from build123d import *

# Parameters (mm, degrees)
F0_R     = 1.5
F1_DEPTH = 1
F4_DEPTH = 66.75
F5_DEPTH = 1


with BuildPart() as f1:
    # F0 (on Top) → F1 (new body)
    with BuildSketch(Plane.XY):
        with BuildLine():
            ThreePointArc((-29, 10.75), (-30.767766953, 10.017766953), (-31.5, 8.25))
            Line((-31.5, 8.25), (-31.5, -8.25))
            ThreePointArc((-31.5, -8.25), (-30.767766953, -10.017766953), (-29, -10.75))
            Line((-29, -10.75), (-22.5, -10.75))
            Line((-22.5, -10.75), (-22.5, 10.75))
            Line((-22.5, 10.75), (-29, 10.75))
        make_face()
        with Locations((-27, -7.625)):
            Circle(F0_R, mode=Mode.SUBTRACT)
        with Locations((-27, 7.625)):
            Circle(F0_R, mode=Mode.SUBTRACT)
    extrude(amount=F1_DEPTH)



with BuildPart() as f1b:
    # F0 (on Top) → F1, piece 2 (new body)
    with BuildSketch(Plane.XY):
        with BuildLine():
            Line((29, 10.75), (22.5, 10.75))
            Line((22.5, 10.75), (22.5, -10.75))
            Line((22.5, -10.75), (29, -10.75))
            ThreePointArc((29, -10.75), (30.767766953, -10.017766953), (31.5, -8.25))
            Line((31.5, -8.25), (31.5, 8.25))
            ThreePointArc((31.5, 8.25), (30.767766953, 10.017766953), (29, 10.75))
        make_face()
        with Locations((27, -7.625)):
            Circle(F0_R, mode=Mode.SUBTRACT)
        with Locations((27, 7.625)):
            Circle(F0_R, mode=Mode.SUBTRACT)
    extrude(amount=F1_DEPTH)


with BuildPart() as f1_1:
    add(f1.part)

    add(f1b.part)  # F4 merges F1b
    # F3 (on offset) → F4 (join)
    with BuildSketch(Plane(origin=(0, 0, -11.5), x_dir=(1, 0, 0), z_dir=(0, 0, -1))):
        Polygon((-22.5, 10.75), (-22.5, -10.75), (-22.5, -15.75), (22.5, -15.75), (22.5, -10.75), (22.5, 10.75), (22.5, 15.75), (-22.5, 15.75), align=None)
        Polygon((-21.5, -14.75), (-21.5, -10.75), (-21.5, 10.75), (-21.5, 14.75), (21.5, 14.75), (21.5, 10.75), (21.5, -10.75), (21.5, -14.75), (8, -14.75), (-8, -14.75), align=None, mode=Mode.SUBTRACT)
    extrude(amount=-F4_DEPTH)

    # F3 (on offset) → F5 (join)
    with BuildSketch(Plane(origin=(0, 0, -11.5), x_dir=(1, 0, 0), z_dir=(0, 0, -1))):
        with BuildLine():
            Line((-21.5, 10.75), (-21.5, -10.75))
            Line((-21.5, -10.75), (-21.5, -14.75))
            Line((-21.5, -14.75), (-8, -14.75))
            Line((-8, -14.75), (-8, 0))
            ThreePointArc((-8, 0), (0, 8), (8, 0))
            Line((8, 0), (8, -14.75))
            Line((8, -14.75), (21.5, -14.75))
            Line((21.5, -14.75), (21.5, -10.75))
            Line((21.5, -10.75), (21.5, 10.75))
            Line((21.5, 10.75), (21.5, 14.75))
            Line((21.5, 14.75), (-21.5, 14.75))
            Line((-21.5, 14.75), (-21.5, 10.75))
        make_face()
    extrude(amount=-F5_DEPTH)


solid = f1_1.part
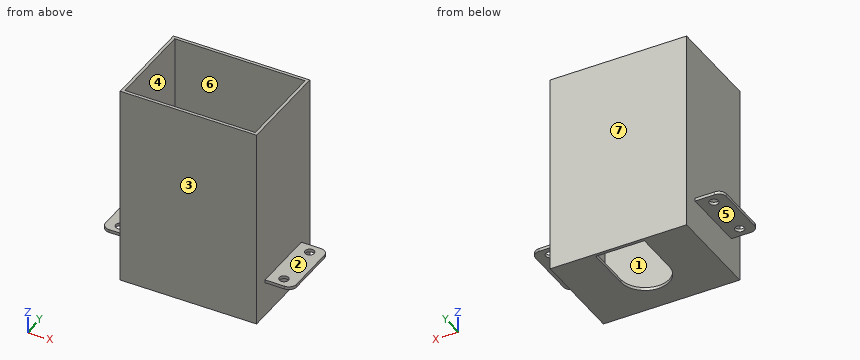
Source: CAD feature listing. Evaluate the final solid. Frame: model axes, mm. Face numbers are marked on the shaded views. A direction names the side the tool comes from. Coordinates: 2 decimals unless noted, no trailing zeros. Loops run counter-clockwise (first coordinate to the right, second up) from the corner with the lowest first, then second, coordinate; pieces in that order, holes last. Notation, with made-up numbers: (68.25, -18.5) - (111.25, -18.5) arc R22 cw to (111.25, 8.5) - close; hole circle Ø3 at (41, 9). An arc over 180 degrees is marked (long way). Return JSON: item names as keys, results as strings.
Q1. Material intervals for line 1 along Y through (x, z) = (27, 0.3) (3 decimals); line 2 along Y through (x, z) = (18.5, 26.5); line 3 along X through (y, z) = (-11.5, 35.5), sorted ascending.
Results:
{"line 1": "-10.75 to -9.125, -6.125 to 6.125, 9.125 to 10.75", "line 2": "-15.75 to -14.75, 14.75 to 15.75", "line 3": "-22.5 to -21.5, 21.5 to 22.5"}
Q2. Contact query for flat-ended pins moving along their axis: P1, Ø7, axis at x = 28.5, y = 3.5, coming from the -Z side; P2, Ø10, axis at y = 6.5, z = 32.5, coming from the +X side; P3, Ø9, axis at y = -2, z = 15.5, coming from the -X side. Output: stop coordinate, or through.
Results:
{"P1": "z = 0", "P2": "x = 22.5", "P3": "x = -22.5"}
Q3. Mould query, pull axis Y, two halves, no side actions, for the marked faces 1, 2, 3 and 4. Classes: released by +Y, released by -Y, zero draft, split by the parting line, or undercut.
Results:
{"face 1": "undercut", "face 2": "zero draft", "face 3": "released by -Y", "face 4": "undercut"}
Q4. Section D-D, the plane x = 18. Return loops of the section in (y, z), plus the area to 3 significant figures.
Results:
{"outline": "(-15.75, -11.5) - (15.75, -11.5) - (15.75, 55.25) - (14.75, 55.25) - (14.75, -10.5) - (-14.75, -10.5) - (-14.75, 55.25) - (-15.75, 55.25) - close", "area": "163 mm2"}
Q5. Section C-C, the plane x = -27. Return loops of the section in (y, z) (3 decimals).
Results:
{"outline": "(-10.75, 0) - (-9.125, 0) - (-9.125, 1) - (-10.75, 1) - close; (-6.125, 0) - (6.125, 0) - (6.125, 1) - (-6.125, 1) - close; (9.125, 0) - (10.75, 0) - (10.75, 1) - (9.125, 1) - close"}
Q6. Section B-B, the plane z = -6. Return loops of the section in (x, y).
Results:
{"outline": "(-22.5, -15.75) - (22.5, -15.75) - (22.5, 15.75) - (-22.5, 15.75) - close; hole (-21.5, -14.75) - (21.5, -14.75) - (21.5, 14.75) - (-21.5, 14.75) - close"}
Q7. Access query for the marked faces 5, 6 and 7. Directions: +Z, -Z, +X, -X, +Y, -Y. A direction counts if a zero-diameter tool reaches every point of the face in a straight line with its end or side. Return the directions, or none.
Results:
{"face 5": "-Z, -X, +Y, -Y", "face 6": "+Z", "face 7": "+Z, -Z, +X, -X, +Y"}
Q8. Section A-A, the plane x = 0. Return loops of the section in (y, z).
Results:
{"outline": "(-15.75, -11.5) - (-8, -11.5) - (-8, -10.5) - (-14.75, -10.5) - (-14.75, 55.25) - (-15.75, 55.25) - close; (14.75, -11.5) - (15.75, -11.5) - (15.75, 55.25) - (14.75, 55.25) - close"}
